from build123d import *

# Parameters (mm, degrees)
F1_DEPTH = 3.175
F2_W     = 86.641395
F2_H     = 19.05
F3_DEPTH = 25.4


with BuildPart() as f1:
    # F0 (on Front) → F1 (new body)
    with BuildSketch(Plane.XZ):
        Polygon((146.05, 325.4375), (0, 325.4375), (0, 0), (279.4, 0), (279.4, 111.125), (146.05, 111.125), align=None)
    extrude(amount=F1_DEPTH)

    # F2 (on face) → F3 (cut)
    with BuildSketch(Plane.XZ.offset(3.175)):
        with BuildLine():
            ThreePointArc((221.7383, 26.608702), (230.341469, 39.484254), (233.3625, 54.672003))
            ThreePointArc((233.3625, 54.672003), (230.341469, 69.859752), (221.7383, 82.735303))
            Line((221.7383, 82.735303), (193.675, 54.672003))
            Line((193.675, 54.672003), (221.7383, 26.608702))
        make_face()
        with BuildLine():
            ThreePointArc((227.061696, 23.241106), (225.854349, 25.04803), (223.722937, 24.624066))
            ThreePointArc((223.722937, 24.624066), (224.357444, 21.434183), (227.061696, 23.241106))
        make_face()
        with BuildLine():
            ThreePointArc((164.199904, 23.241106), (164.051027, 23.989559), (163.627063, 24.624066))
            ThreePointArc((163.627063, 24.624066), (160.43718, 22.492654), (164.199904, 23.241106))
        make_face()
        with BuildLine():
            ThreePointArc((164.199904, 86.102899), (160.43718, 86.851352), (163.627063, 84.71994))
            ThreePointArc((163.627063, 84.71994), (164.051027, 85.354447), (164.199904, 86.102899))
        make_face()
        with BuildLine():
            ThreePointArc((227.061696, 86.102899), (224.357444, 87.909823), (223.722937, 84.71994))
            ThreePointArc((223.722937, 84.71994), (225.854349, 84.295976), (227.061696, 86.102899))
        make_face()
        with BuildLine():
            Line((193.675, 54.672003), (221.7383, 82.735303))
            ThreePointArc((221.7383, 82.735303), (193.675, 94.359503), (165.6117, 82.735303))
            Line((165.6117, 82.735303), (193.675, 54.672003))
        make_face()
        with BuildLine():
            ThreePointArc((165.6117, 26.608702), (193.675, 14.984503), (221.7383, 26.608702))
            Line((221.7383, 26.608702), (193.675, 54.672003))
            Line((193.675, 54.672003), (165.6117, 26.608702))
        make_face()
        with BuildLine():
            Line((193.675, 54.672003), (165.6117, 82.735303))
            ThreePointArc((165.6117, 82.735303), (153.9875, 54.672003), (165.6117, 26.608702))
            Line((165.6117, 26.608702), (193.675, 54.672003))
        make_face()
        with BuildLine():
            ThreePointArc((36.62532, 211.02468), (40.066588, 216.174901), (41.275, 222.25))
            ThreePointArc((41.275, 222.25), (40.066588, 228.325099), (36.62532, 233.47532))
            Line((36.62532, 233.47532), (25.4, 222.25))
            Line((25.4, 222.25), (36.62532, 211.02468))
        make_face()
        with BuildLine():
            ThreePointArc((41.56185, 208.2408), (40.232983, 210.22959), (37.887046, 209.762954))
            ThreePointArc((37.887046, 209.762954), (38.585416, 206.252011), (41.56185, 208.2408))
        make_face()
        with BuildLine():
            ThreePointArc((13.54345, 208.2408), (13.37959, 209.064584), (12.912954, 209.762954))
            ThreePointArc((12.912954, 209.762954), (9.402011, 207.417017), (13.54345, 208.2408))
        make_face()
        with BuildLine():
            ThreePointArc((13.54345, 236.2592), (9.402011, 237.082983), (12.912954, 234.737046))
            ThreePointArc((12.912954, 234.737046), (13.37959, 235.435416), (13.54345, 236.2592))
        make_face()
        with BuildLine():
            ThreePointArc((41.56185, 236.2592), (38.585416, 238.247989), (37.887046, 234.737046))
            ThreePointArc((37.887046, 234.737046), (40.232983, 234.27041), (41.56185, 236.2592))
        make_face()
        with BuildLine():
            Line((25.4, 222.25), (36.62532, 233.47532))
            ThreePointArc((36.62532, 233.47532), (25.4, 238.125), (14.17468, 233.47532))
            Line((14.17468, 233.47532), (25.4, 222.25))
        make_face()
        with BuildLine():
            ThreePointArc((14.17468, 211.02468), (25.4, 206.375), (36.62532, 211.02468))
            Line((36.62532, 211.02468), (25.4, 222.25))
            Line((25.4, 222.25), (14.17468, 211.02468))
        make_face()
        with BuildLine():
            Line((25.4, 222.25), (14.17468, 233.47532))
            ThreePointArc((14.17468, 233.47532), (9.525, 222.25), (14.17468, 211.02468))
            Line((14.17468, 211.02468), (25.4, 222.25))
        make_face()
        with BuildLine():
            ThreePointArc((120.54389, 260.696076), (126.911611, 270.226044), (129.147658, 281.467408))
            ThreePointArc((129.147658, 281.467408), (126.911611, 292.708772), (120.54389, 302.23874))
            Line((120.54389, 302.23874), (99.772558, 281.467408))
            Line((99.772558, 281.467408), (120.54389, 260.696076))
        make_face()
        with BuildLine():
            ThreePointArc((125.49838, 257.894236), (124.169513, 259.883025), (121.823577, 259.416389))
            ThreePointArc((121.823577, 259.416389), (122.521946, 255.905446), (125.49838, 257.894236))
        make_face()
        with BuildLine():
            ThreePointArc((78.352035, 257.894236), (78.188175, 258.718019), (77.721539, 259.416389))
            ThreePointArc((77.721539, 259.416389), (74.210596, 257.070452), (78.352035, 257.894236))
        make_face()
        with BuildLine():
            ThreePointArc((78.352035, 305.04058), (74.210596, 305.864364), (77.721539, 303.518427))
            ThreePointArc((77.721539, 303.518427), (78.188175, 304.216797), (78.352035, 305.04058))
        make_face()
        with BuildLine():
            ThreePointArc((125.49838, 305.04058), (122.521946, 307.02937), (121.823577, 303.518427))
            ThreePointArc((121.823577, 303.518427), (124.169513, 303.051791), (125.49838, 305.04058))
        make_face()
        with BuildLine():
            Line((99.772558, 281.467408), (120.54389, 302.23874))
            ThreePointArc((120.54389, 302.23874), (99.772558, 310.842508), (79.001225, 302.23874))
            Line((79.001225, 302.23874), (99.772558, 281.467408))
        make_face()
        with BuildLine():
            ThreePointArc((79.001225, 260.696076), (99.772558, 252.092308), (120.54389, 260.696076))
            Line((120.54389, 260.696076), (99.772558, 281.467408))
            Line((99.772558, 281.467408), (79.001225, 260.696076))
        make_face()
        with BuildLine():
            Line((99.772558, 281.467408), (79.001225, 302.23874))
            ThreePointArc((79.001225, 302.23874), (70.397458, 281.467408), (79.001225, 260.696076))
            Line((79.001225, 260.696076), (99.772558, 281.467408))
        make_face()
        with Locations((68.720697, 158.75)):
            Rectangle(F2_W, F2_H)
        with Locations((68.720697, 123.825)):
            Rectangle(F2_W, F2_H)
        with BuildLine():
            ThreePointArc((98.559112, 33.90067), (104.926833, 43.430639), (107.162879, 54.672003))
            ThreePointArc((107.162879, 54.672003), (104.926833, 65.913367), (98.559112, 75.443335))
            Line((98.559112, 75.443335), (77.787779, 54.672003))
            Line((77.787779, 54.672003), (98.559112, 33.90067))
        make_face()
        with BuildLine():
            ThreePointArc((103.513602, 31.098831), (102.184735, 33.08762), (99.838798, 32.620984))
            ThreePointArc((99.838798, 32.620984), (100.537168, 29.110041), (103.513602, 31.098831))
        make_face()
        with BuildLine():
            ThreePointArc((56.367257, 31.098831), (56.203396, 31.922614), (55.73676, 32.620984))
            ThreePointArc((55.73676, 32.620984), (52.225818, 30.275047), (56.367257, 31.098831))
        make_face()
        with BuildLine():
            ThreePointArc((56.367257, 78.245175), (52.225818, 79.068959), (55.73676, 76.723022))
            ThreePointArc((55.73676, 76.723022), (56.203396, 77.421392), (56.367257, 78.245175))
        make_face()
        with BuildLine():
            ThreePointArc((103.513602, 78.245175), (100.537168, 80.233964), (99.838798, 76.723022))
            ThreePointArc((99.838798, 76.723022), (102.184735, 76.256386), (103.513602, 78.245175))
        make_face()
        with BuildLine():
            Line((77.787779, 54.672003), (98.559112, 75.443335))
            ThreePointArc((98.559112, 75.443335), (77.787779, 84.047103), (57.016447, 75.443335))
            Line((57.016447, 75.443335), (77.787779, 54.672003))
        make_face()
        with BuildLine():
            ThreePointArc((57.016447, 33.90067), (77.787779, 25.296903), (98.559112, 33.90067))
            Line((98.559112, 33.90067), (77.787779, 54.672003))
            Line((77.787779, 54.672003), (57.016447, 33.90067))
        make_face()
        with BuildLine():
            Line((77.787779, 54.672003), (57.016447, 75.443335))
            ThreePointArc((57.016447, 75.443335), (48.412679, 54.672003), (57.016447, 33.90067))
            Line((57.016447, 33.90067), (77.787779, 54.672003))
        make_face()
    extrude(amount=-F3_DEPTH, mode=Mode.SUBTRACT)


solid = f1.part
Read the model definition and answer for the solid it produces. Units are mm, in the model's axes. Round coordinates to 2 decimals unless told otherwise and drop trailing zeros. Order: outer loops, then holes, each group sorted by start corner. A loop starts at its lowest first (then second) coordinate and runs counter-clockwise, first axis right, second up. Notation, with made-up numbers: (88, -10) - (126, -10) arc R36 ccw to (126, 24) - close; hole circle Ø9 at (-3, -25.5). An arc over 180 degrees is marked (long way). Use one line per item in the form item = value. Start each with the question number.
(1) Flat-ended cylindrical pins translate along their axes: pin 1 Ø2 at (x, z) = (155, 60) entering from -Y (3 decimals); pin 2 Ø3 at (x, z) = (162.24, 23.24) entering from -Y. Find the tip coordinate at first contact, or state that the pin passes through.
(2) The part is cut by section C-C (x = 66). Count the separate pieces of the cut face and the enclosed holes in it, then the cut area to 3 significant figures.
(3) The part is cut by section A-A (z = 128). Give the vertices of the cut face in (x, y) (3 decimals), then the cut area to 3 significant figures.
(4) Find the intervals of material crossed by line 1 along X through (y, z) = (-0.5, 155); line 2 along X through (y, z) = (-1.45, 86); line 3 along Z through (x, y) = (236.5, -1.45) (3 decimals), in increasing order. Write a range as from..to.
(5) The part is cut by section B-B (x = 203). Give the vertices of the cut face in (y, z) (3 decimals).
Checked values:
q1.pin_1 = -3.175
q1.pin_2 = through
q2.separate_pieces = 4
q2.enclosed_holes = 0
q2.area = 741 mm^2
q3.outline = (0, -3.175) - (25.4, -3.175) - (25.4, 0) - (0, 0) - close; (112.041, -3.175) - (146.05, -3.175) - (146.05, 0) - (112.041, 0) - close
q3.area = 189 mm^2
q4.line_1 = 0..25.4, 112.04..146.05
q4.line_2 = 0..160.29, 164.2..169.31, 218.04..223.15, 227.06..279.4
q4.line_3 = 0..111.125
q5.outline = (-3.175, 0) - (0, 0) - (0, 16.096) - (-3.175, 16.096) - close; (-3.175, 93.248) - (0, 93.248) - (0, 111.125) - (-3.175, 111.125) - close
